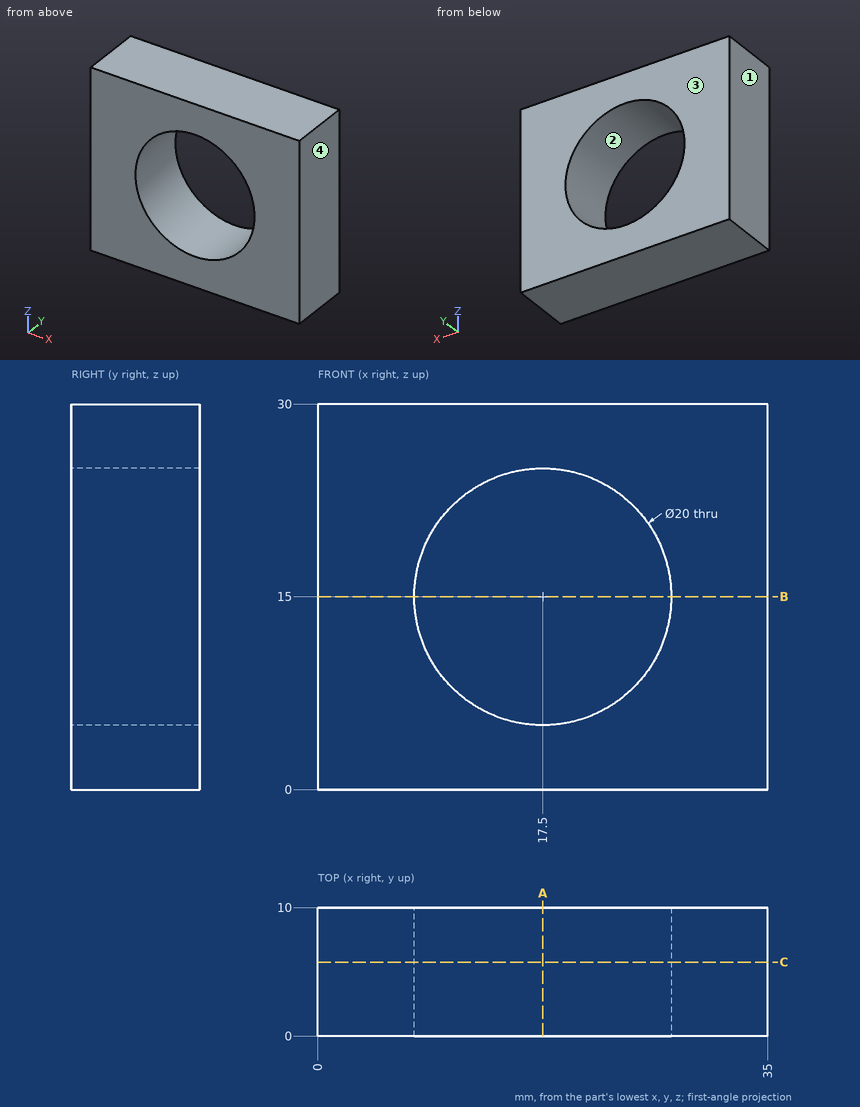
Design review of the part shown in the three views and the two pictorial views. Dimensions are in mm from the part's minimum x, y and z. Round coordinates to 2 decimals unless told otherwise and drop trailing zeros. Loops run counter-clockwise (first coordinate to the right, second up) from the corner with the lowest first, then second, coordinate; pieces in that order, holes last. Notation, with made-up numbers: M 25,86 L 69,86 A11 cw 69,98 Z; hole C -4.75,-19 d1. An arc over 180 degrees is marked long. Answer as a JSON object with one key per item and string values.
Item 1: We need section A-A on x = 17.5. Give the boundary of the cut face in (y, z).
Answer sheet:
{"outline": "M 0,0 L 10,0 L 10,5 L 0,5 Z; M 0,25 L 10,25 L 10,30 L 0,30 Z"}
Item 2: Wall thickness on L1, parallel to Z at x = 17.5, y = 6.25; L2, parallel to X at y = 3, z = 6; L3, parallel to Z at x = 21, y = 7.75: over which ranges is each line inside the solid? List them lowest first. Write a range as from..to.
Answer sheet:
{"L1": "z = 0..5, 25..30", "L2": "x = 0..13.14, 21.86..35", "L3": "z = 0..5.63, 24.37..30"}
Item 3: We need section C-C on y = 5.75. Give the boundary of the cut face in (x, z).
Answer sheet:
{"outline": "M 0,0 L 35,0 L 35,30 L 0,30 Z; hole C 17.5,15 d20"}
Item 4: Clearance check with a flat-ended pin moving along its axis: P1, Ø2, axis at x = 25, z = 19, coming from the -Y side. State where the tip first meets the part, or that it passes through.
Answer sheet:
{"P1": "passes through"}
Item 5: The part is to be moulded in two halves that separate along X. For the marked faces 1, 2, 3 and 4, say which applies: pulls with the +X half, pulls with the -X half, needs draft (parallel to the pull), parting line crosses it, or undercut.
Answer sheet:
{"face 1": "pulls with the -X half", "face 2": "undercut", "face 3": "needs draft", "face 4": "pulls with the +X half"}
Item 6: We need section B-B on z = 15. Give the boundary of the cut face in (x, y).
Answer sheet:
{"outline": "M 0,0 L 7.5,0 L 7.5,10 L 0,10 Z; M 27.5,0 L 35,0 L 35,10 L 27.5,10 Z"}
